from build123d import *

# Parameters (mm, degrees)
F0_W     = 50.8
F0_H     = 2.54
F1_DEPTH = 152.4
F2_W     = 12.7
F2_H     = 152.4
F3_DEPTH = 50.8
F4_W     = 38.1
F4_H     = 7.62
F5_DEPTH = 50.8
F6_DEPTH = 50.8
F7_W     = 10.16
F7_H     = 137.16
F8_DEPTH = 10.16


with BuildPart() as f1:
    # F0 (on Front) → F1 (new body)
    with BuildSketch(Plane.XZ):
        with Locations((-36.653862, 12.186867)):
            Rectangle(F0_W, F0_H)
    extrude(amount=F1_DEPTH)

    # F2 (on face) → F3 (join)
    with BuildSketch(Plane.XY.offset(13.456867)):
        with Locations((-55.703862, -76.2)):
            Rectangle(F2_W, F2_H)
    extrude(amount=F3_DEPTH)

    # F4 (on face) → F5 (join)
    with BuildSketch(Plane.XY.offset(13.456867)):
        with Locations((-30.303862, -148.59)):
            Rectangle(F4_W, F4_H)
    extrude(amount=F5_DEPTH)

    # F4 (on face) → F6 (join)
    with BuildSketch(Plane.XY.offset(13.456867)):
        with Locations((-30.303862, -3.81)):
            Rectangle(F4_W, F4_H)
    extrude(amount=F6_DEPTH)

    # F7 (on face) → F8 (join)
    with BuildSketch(Plane.XY.offset(13.456867)):
        with Locations((-16.333862, -76.2)):
            Rectangle(F7_W, F7_H)
    extrude(amount=F8_DEPTH)


solid = f1.part
Input: part model. Units: mm. Frame: model coordinates. A direction names the side the tool comes from. Round coordinates to 2 decimals unless told otherwise and drop trailing zeros. Loops run counter-clockwise (first coordinate to the right, second up) from the corner with the lowest first, then second, coordinate; pieces in that order, holes last. Notation, with made-up numbers: M 59,-11.75 L 72,-11.75 A11 ccw 72,3.25 Z; hole C -36.5,40 d11. An arc over 180 degrees is marked long. Answer as CSV lines item,"result". Start each with the question number.
(1) Section A-A, the plane z = 53. Output: boundary loops of the cut face in (x, y).
(2) Line query: line 1 (Y direction, x = -34, z = 16.5); line 2 (Z direction, x = -31, y = -119); line 3 (X direction, y = -65, z = 60). Output: solid intervals per line, ascending. Write a range as [from, to].
(3) Reachability of faces 4 (the flat face through (-16, -75, 23.617)), 5 (the flat face through (-62.054, -77, 37)), 6 (the flat face through (-31, -144.78, 39)) from +Z, -Z, +X, -X, +Y, -Y: full face, straight path, thin tool, end or side. Return the list, or none.
(4) Section C-C, the plane x = -30. Output: boundary loops of the cut face in (y, z).
(5) First-contact query: pin 1 (3 mm diameter, centred on y = -68.5, z = 36.5, fed in from +X); pin 2 (11.5 mm diameter, centred on x = -37, z = 27.5, fed in from +Y); pin 3 (1 mm diameter, centred on x = -27.5, y = -106.5, fed in from +Z); pin 4 (8 mm diameter, centred on x = -16, y = -67, fed in from +Z). Flat tips, straight axial feed; report the tip coordinate or a pass-through.
(6) Section B-B, the plane z = 21. Output: boundary loops of the cut face in (x, y), plus the area to 3 significant figures.
(7) Draft query along X for faces 1 (the flat face through (-52, -76, 64.257)), 2 (the flat face through (-36, -75, 13.457)), 3 (the flat face through (-11.254, -77, 20)). Return one class per face: released by +X, released by -X, zero draft, split by the parting line, or undercut.
Values found:
1,outline,"M -62.05,-152.4 L -11.25,-152.4 L -11.25,-144.78 L -49.35,-144.78 L -49.35,-7.62 L -11.25,-7.62 L -11.25,0 L -62.05,0 Z"
2,line 1,"y = [-152.4, -144.78], [-7.62, 0]"
2,line 2,"z = [10.92, 13.46]"
2,line 3,"x = [-62.05, -49.35]"
3,face 4,"+Z, +X"
3,face 5,"+Z, -Z, -X, +Y, -Y"
3,face 6,"+Z"
4,outline,"M -152.4,10.92 L 0,10.92 L 0,64.26 L -7.62,64.26 L -7.62,13.46 L -144.78,13.46 L -144.78,64.26 L -152.4,64.26 Z"
5,pin 1,"stops at x = -49.35"
5,pin 2,"stops at y = 0"
5,pin 3,"stops at z = 13.46"
5,pin 4,"stops at z = 23.62"
6,outline,"M -62.05,-152.4 L -11.25,-152.4 L -11.25,0 L -62.05,0 Z; hole M -49.35,-144.78 L -21.41,-144.78 L -21.41,-7.62 L -49.35,-7.62 Z"
6,area,"3,910 mm²"
7,face 1,"zero draft"
7,face 2,"undercut"
7,face 3,"released by +X"
